The listing builds one solid part. Answer for the finished solid, in the listing's coordinates (mm). A direction names the side the tool comes from. Coordinates: 2 decimals unless noted, no trailing zeros. Write each loop counter-clockwise with the first axis right and the second up, starting at its lowest first coordinate (ties: lowest second). Pieces come first, ordered by that corner, then holes. Notation, with made-up numbers: M -31,-26.5 L 8,-26.5 A18 ccw 8,-3.5 Z; hole C 29.5,66.25 d3. An arc over 180 degrees is marked long. Answer as CSV lines item,"result". Start each with the question number.
Autodesk Inventor part; units mm, degrees
ref_plane "YZ Plane" through (0, 0, 0) normal (1, 0, 0) x (0, 1, 0)
ref_plane "XZ Plane" through (0, 0, 0) normal (0, 1, 0) x (-1, 0, 0)
ref_plane "XY Plane" through (0, 0, 0) normal (0, 0, 1) x (1, 0, 0)
sketch "Esquisse1" plane through (0, 0, 0) normal (0, 0, 1) x (1, 0, 0)
  circle A0 centre (0, 0) radius 25
  point P0 (0, -25)
  point P1 (0, 25)
  dimension "d0" = 50
extrude "Extrusion1" add sketch "Esquisse1" along normal blind 200
sketch "Esquisse2" plane through (0, 0, 0) normal (0, 0, -1) x (-1, 0, 0)
  point P0 (0, 0)
sketch "Esquisse3" plane through (0, 0, 200) normal (0, 0, 1) x (1, 0, 0)
  circle A0 centre (0, 0) radius 25
  point P0 (0, -25)
ref_plane "Plan de construction1" through (0, -25, 0) normal (1, 0, 0) x (0, 1, 0)
sketch "Esquisse4" plane through (0, -25, 0) normal (1, 0, 0) x (0, 1, 0)
  line L0 (-175, -400) -> (225, -400)
  line L1 (225, -400) -> (225, 0)
  line L2 (225, 0) -> (-175, 0)
  line L3 (-175, 0) -> (-175, -400)
  line L4 (0, 0) -> (50, 0)
  line L5 (-140, -365) -> (190, -365)
  line L6 (190, -365) -> (190, -35)
  line L7 (190, -35) -> (-140, -35)
  line L8 (-140, -35) -> (-140, -365)
  point P0 (25, 0)
  dimension "d3" = 0
  dimension "d4" = 400
  dimension "d5" = 400
  dimension "d6" = 200
  dimension "d7" = 330
  dimension "d8" = 330
  dimension "d9" = 35
  dimension "d10" = 35
extrude "Extrusion2" add sketch "Esquisse4" along normal mid plane 20
ref_plane "Plan de construction2" through (0, 0, 100) normal (0, 0, 1) x (1, 0, 0)
sketch "Esquisse5" plane through (0, 0, 100) normal (0, 0, 1) x (1, 0, 0)
  circle A0 centre (0, 0) radius 25
equation "\"d9\" = -0.5 * d8 + 0.5 * d5"
equation "\"d10\" = -0.5 * d8 + 0.5 * d5"
properties part number "raquetteEsquisse" material "Plastique ABS"
1) The part is cut by section D-D (y = 0). Determine the outline of the cut face in (x, z).
2) Find the intervals of material crossed by line 1 (Y direction, x = -7, z = -312.5); line 2 (Z direction, x = 1, y = -63); line 3 (Y direction, x = -2, z = 14), in increasing order. Write a range as from..to.
3) For a pull along Z with two mould halves and no side action, classify faces 1 (the face through (0, -2, -365)), 2 (the face through (16, 0, 0)), 3 (the face through (-10, -181, -197)) as +Z half, -Z half, draft (parallel to the pull), parting line (faces both ways), or undercut.
4) Which of the six approach directions +Z, -Z, +X, -X, +Y, -Y give full straight-line access (tool end or side, diameter ignored) to faces 4 (the face through (0, -3, -400)), 5 (the face through (23.846, -7.509, 98.6)), 6 (the face through (0, 165, -202)), 7 (the face through (-16, 0, 0)), 8 (the face through (0, 0, 200))?
5) The part is cut by section B-B (y = -125.5). Determine the outline of the cut face in (x, z).
6) The part is cut by section C-C (x = 0). Determine the outline of the cut face in (y, z), then the cut area to 3 significant figures.
7) Each of these flat-tipped pins is pushed along its axis until it touches: P1, Ø3, axis at x = -6, z = 90, coming from the +Y side; P2, Ø4.5, axis at x = 19.5, y = 10.5, coming from the -Z side; P3, Ø22, axis at x = 0.5, y = 81, coming from the +Z side. Where does it stop, or does it pass through?
8) The part is cut by section A-A (z = -150.5). Determine the outline of the cut face in (x, y), then the cut area to 3 significant figures.
Completed:
1,outline,"M -25,0 L -10,0 L -10,-35 L 10,-35 L 10,0 L 25,0 L 25,200 L -25,200 Z; M -10,-400 L 10,-400 L 10,-365 L -10,-365 Z"
2,line 1,"-200..-165, 165..200"
2,line 2,"-400..-365, -35..0"
2,line 3,"-24.92..24.92"
3,face 1,"undercut"
3,face 2,"-Z half"
3,face 3,"draft"
4,face 4,"-Z, +X, -X, +Y, -Y"
4,face 5,"+Z"
4,face 6,"+X, -X"
4,face 7,"-Z, -X, +Y, -Y"
4,face 8,"+Z, +X, -X, +Y, -Y"
5,outline,"M -10,-400 L 10,-400 L 10,-365 L -10,-365 Z; M -10,-35 L 10,-35 L 10,0 L -10,0 Z"
6,outline,"M -200,-400 L 200,-400 L 200,0 L 25,0 L 25,200 L -25,200 L -25,0 L -200,0 Z; hole M -165,-365 L 165,-365 L 165,-35 L -165,-35 Z"
6,area,"61,100 mm²"
7,P1,"y = 24.59"
7,P2,"z = 0"
7,P3,"z = 0"
8,outline,"M -10,-200 L 10,-200 L 10,-165 L -10,-165 Z; M -10,165 L 10,165 L 10,200 L -10,200 Z"
8,area,"1,400 mm²"
